Here's how the part is built. I have some questions about the finished solid (model axes, mm). Face numbers are marked on the shaded views. A direction names the side the tool comes from. Round coordinates to 2 decimals unless told otherwise and drop trailing zeros. Write each loop counter-clockwise with the first axis right and the second up, starting at its lowest first coordinate (ties: lowest second). Pieces come first, ordered by that corner, then holes. Notation, with made-up numbers: (74, 31) -> (94, 31) arc R10 ccw to (94, 41) -> close; hole circle Ø6 at (-33, 12). An arc over 180 degrees is marked (long way). Put each result on its own line as item: value. Start each with the question number.
1) Will these pins go through, and if not, where does the flat tip stop? P1, Ø5, axis at x = 95.5, z = 20.5, coming from the +Y side; P2, Ø12, axis at y = 18.5, z = 44.5, coming from the -X side; P3, Ø3, axis at y = 36, z = -29.5, coming from the +X side.
2) Which directions (+Z, -Z, +X, -X, +Y, -Y) give clear straight access to the entire face, cutting with the end or side of a thin tool? Please do the marked faces 1, 2 and 3.
3) If I drill on line 1 along X through (y, z) = (1.4, 40); line 2 along X through (y, z) = (35, -19), over which ranges is the centre line in solid material (lowest first)? Write a range as [from, to].
4) I want a section at D-D, the plane z = -6.5. List the corners of the cut face in (x, y) for me.
5) I want a section at B-B, the plane x = -96. List the corners of the cut face in (y, z) for me, then the cut area to 3 significant figures.
6) I want a section at A-A, the plane z = -40. List the corners of the cut face in (x, y) for me.
7) I want a section at C-C, the plane y = 37. List the corners of the cut face in (x, z) for me.
from build123d import *

# Parameters (mm, degrees)
SKETCH_2_W      = 205
SKETCH_2_H      = 127
SKETCH_2_R      = 2
EXTRUDE_1_DEPTH = 3
SKETCH_3_W      = 177
SKETCH_3_H      = 127
EXTRUDE_2_DEPTH = 52
FILLET_1_R      = 2


with BuildPart() as part:
    # 草图2 → 凸台-拉伸1 (new body)
    with BuildSketch(Plane(origin=(0, 0, 0), x_dir=(1, 0, 0), z_dir=(0, 1, 0))):
        Rectangle(SKETCH_2_W, SKETCH_2_H)
        with Locations(Location((-96, 40, 0), (0, 0, 270))):
            Circle(SKETCH_2_R, mode=Mode.SUBTRACT)
        with Locations(Location((96, 40, 0), (0, 0, 270))):
            Circle(SKETCH_2_R, mode=Mode.SUBTRACT)
        with Locations(Location((96, -40, 0), (0, 0, 270))):
            Circle(SKETCH_2_R, mode=Mode.SUBTRACT)
        with Locations(Location((-96, -40, 0), (0, 0, 270))):
            Circle(SKETCH_2_R, mode=Mode.SUBTRACT)
    extrude(amount=EXTRUDE_1_DEPTH)

    # 草图3 → 凸台-拉伸2 (add)
    with BuildSketch(Plane(origin=(0, 3, 0), x_dir=(1, 0, 0), z_dir=(0, 1, 0))):
        Rectangle(SKETCH_3_W, SKETCH_3_H)
    extrude(amount=EXTRUDE_2_DEPTH)

    # 圆角1
    fillet_1_edges = [part.edges().sort_by_distance(p)[0] for p in [
        (-88.5, 29, 63.5),
        (88.5, 29, 63.5),
        (88.5, 29, -63.5),
        (-88.5, 55, 0),
        (0, 55, 63.5),
        (88.5, 55, 0),
        (0, 55, -63.5),
    ]]
    fillet(fillet_1_edges, radius=FILLET_1_R)


solid = part.part
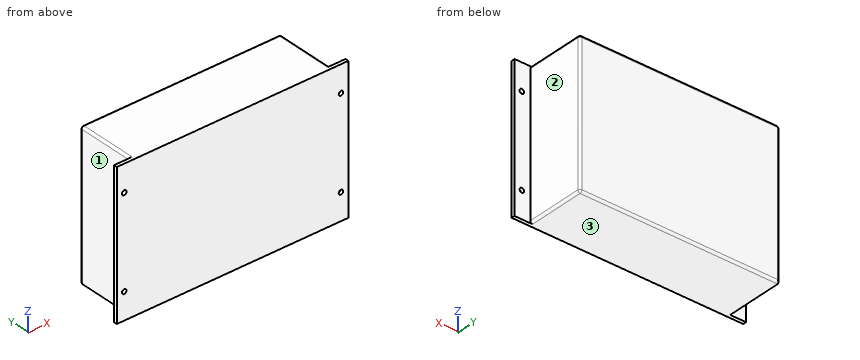
Findings:
1. P1: stops at y = 3
1. P2: stops at x = -88.5
1. P3: stops at x = 88.5
2. face 1: +Z, -Z, -X, +Y
2. face 2: +Z, -Z, +X, +Y
2. face 3: -Z, +X, -X, +Y, -Y
3. line 1: x = [-102.5, -98], [-94, 94], [98, 102.5]
3. line 2: x = [-88.5, 88.5]
4. outline: (-102.5, 0) -> (102.5, 0) -> (102.5, 3) -> (88.5, 3) -> (88.5, 53) arc R2 ccw to (86.5, 55) -> (-86.5, 55) arc R2 ccw to (-88.5, 53) -> (-88.5, 3) -> (-102.5, 3) -> close
5. outline: (0, -63.5) -> (3, -63.5) -> (3, -42) -> (0, -42) -> close; (0, -38) -> (3, -38) -> (3, 38) -> (0, 38) -> close; (0, 42) -> (3, 42) -> (3, 63.5) -> (0, 63.5) -> close
5. area: 357 mm2
6. outline: (-102.5, 0) -> (-98, 0) -> (-98, 3) -> (-102.5, 3) -> close; (-94, 0) -> (94, 0) -> (94, 3) -> (88.5, 3) -> (88.5, 53) arc R2 ccw to (86.5, 55) -> (-86.5, 55) arc R2 ccw to (-88.5, 53) -> (-88.5, 3) -> (-94, 3) -> close; (98, 0) -> (102.5, 0) -> (102.5, 3) -> (98, 3) -> close
7. outline: (-88.5, -63.5) -> (86.5, -63.5) arc R2 ccw to (88.5, -61.5) -> (88.5, 61.5) arc R2 ccw to (86.5, 63.5) -> (-86.5, 63.5) arc R2 ccw to (-88.5, 61.5) -> close
